Design review of the part built by this model. Coordinates are the model's own, in mm. A direction names the side the tool comes from. Round coordinates to 2 decimals unless told otherwise and drop trailing zeros. Order: outer loops, then holes, each group sorted by start corner. A loop starts at its lowest first (then second) coordinate and runs counter-clockwise, first axis right, second up.
from build123d import *

# Parameters (mm, degrees)
F0_W      = 19
F0_H      = 19
F1_DEPTH  = 19
F3_DEPTH  = 1
F4_R      = 1
F5_DEPTH  = 1
F6_R      = 1
F7_DEPTH  = 1
F8_R      = 1
F9_DEPTH  = 1
F10_R     = 1
F11_DEPTH = 1
F12_R     = 1
F13_DEPTH = 1
F14_R     = 1


with BuildPart() as f1:
    # F0 (on Top) → F1 (new body)
    with BuildSketch(Plane.XY):
        with Locations((-9.5, 9.5)):
            Rectangle(F0_W, F0_H)
    extrude(amount=F1_DEPTH)

    # F2 (on face) → F3 (cut)
    with BuildSketch(Plane.XY.offset(19)):
        with BuildLine():
            ThreePointArc((-10.6875, 9.818189666), (-11.556810334, 10.6875), (-11.875, 11.875))
            Line((-11.875, 11.875), (-11.875, 7.125))
            ThreePointArc((-11.875, 7.125), (-11.556810334, 8.3125), (-10.6875, 9.181810334))
            Line((-10.6875, 9.181810334), (-10.6875, 9.818189666))
        make_face()
        with BuildLine():
            ThreePointArc((-10.6875, 13.931810334), (-11.556810334, 13.0625), (-11.875, 11.875))
            ThreePointArc((-11.875, 11.875), (-11.556810334, 10.6875), (-10.6875, 9.818189666))
            Line((-10.6875, 9.818189666), (-10.6875, 11.875))
            Line((-10.6875, 11.875), (-10.6875, 13.931810334))
        make_face()
        with BuildLine():
            ThreePointArc((-7.125, 11.875), (-8.3125, 13.931810334), (-10.6875, 13.931810334))
            Line((-10.6875, 13.931810334), (-10.6875, 11.875))
            Line((-10.6875, 11.875), (-10.6875, 9.818189666))
            ThreePointArc((-10.6875, 9.818189666), (-10.1146952321, 9.5809261626), (-9.5, 9.5))
            ThreePointArc((-9.5, 9.5), (-7.8206213947, 10.1956213947), (-7.125, 11.875))
        make_face()
        with BuildLine():
            ThreePointArc((-8.3125, 11.875), (-9.5, 10.6875), (-10.6875, 11.875))
            ThreePointArc((-10.6875, 11.875), (-9.5, 13.0625), (-8.3125, 11.875))
        make_face(mode=Mode.SUBTRACT)
        with BuildLine():
            ThreePointArc((-9.5, 9.5), (-10.1146952321, 9.4190738374), (-10.6875, 9.181810334))
            Line((-10.6875, 9.181810334), (-10.6875, 7.125))
            Line((-10.6875, 7.125), (-10.6875, 5.068189666))
            ThreePointArc((-10.6875, 5.068189666), (-8.3125, 5.068189666), (-7.125, 7.125))
            ThreePointArc((-7.125, 7.125), (-7.8206213947, 8.8043786053), (-9.5, 9.5))
        make_face()
        with BuildLine():
            ThreePointArc((-8.3125, 7.125), (-9.5, 5.9375), (-10.6875, 7.125))
            ThreePointArc((-10.6875, 7.125), (-9.5, 8.3125), (-8.3125, 7.125))
        make_face(mode=Mode.SUBTRACT)
        with BuildLine():
            ThreePointArc((-10.6875, 9.181810334), (-11.556810334, 8.3125), (-11.875, 7.125))
            ThreePointArc((-11.875, 7.125), (-11.556810334, 5.9375), (-10.6875, 5.068189666))
            Line((-10.6875, 5.068189666), (-10.6875, 7.125))
            Line((-10.6875, 7.125), (-10.6875, 9.181810334))
        make_face()
        with BuildLine():
            ThreePointArc((-9.5, 9.5), (-10.1146952321, 9.5809261626), (-10.6875, 9.818189666))
            Line((-10.6875, 9.818189666), (-10.6875, 9.181810334))
            ThreePointArc((-10.6875, 9.181810334), (-10.1146952321, 9.4190738374), (-9.5, 9.5))
        make_face()
        with BuildLine():
            ThreePointArc((-10.6875, 5.068189666), (-11.556810334, 5.9375), (-11.875, 7.125))
            Line((-11.875, 7.125), (-11.875, 4.75))
            Line((-11.875, 4.75), (-10.6875, 4.75))
            Line((-10.6875, 4.75), (-10.6875, 5.068189666))
        make_face()
        with BuildLine():
            Line((-10.6875, 14.25), (-11.875, 14.25))
            Line((-11.875, 14.25), (-11.875, 11.875))
            ThreePointArc((-11.875, 11.875), (-11.556810334, 13.0625), (-10.6875, 13.931810334))
            Line((-10.6875, 13.931810334), (-10.6875, 14.25))
        make_face()
    extrude(amount=-F3_DEPTH, mode=Mode.SUBTRACT)

    # F4 (on face) → F5 (cut)
    with BuildSketch(Plane.XZ):
        with Locations((-14.25, 14.25)):
            Circle(F4_R)
        with Locations((-4.75, 4.75)):
            Circle(F4_R)
    extrude(amount=-F5_DEPTH, mode=Mode.SUBTRACT)

    # F6 (on face) → F7 (cut)
    with BuildSketch(Plane(origin=(0, 0, 0), x_dir=(1, 0, 0), z_dir=(0, 0, -1))):
        with Locations((-14.25, -4.75)):
            Circle(F6_R)
        with Locations((-9.5, -9.5)):
            Circle(F6_R)
        with Locations((-4.75, -4.75)):
            Circle(F6_R)
        with Locations((-4.75, -14.25)):
            Circle(F6_R)
        with Locations((-14.25, -14.25)):
            Circle(F6_R)
    extrude(amount=-F7_DEPTH, mode=Mode.SUBTRACT)

    # F8 (on face) → F9 (cut)
    with BuildSketch(Plane(origin=(0, 19, 0), x_dir=(-1, 0, 0), z_dir=(0, 1, 0))):
        with Locations((4.75, 14.25)):
            Circle(F8_R)
        with Locations((4.75, 9.5)):
            Circle(F8_R)
        with Locations((4.75, 4.75)):
            Circle(F8_R)
        with Locations((14.25, 4.75)):
            Circle(F8_R)
        with Locations((14.25, 9.5)):
            Circle(F8_R)
        with Locations((14.25, 14.25)):
            Circle(F8_R)
    extrude(amount=-F9_DEPTH, mode=Mode.SUBTRACT)

    # F10 (on face) → F11 (cut)
    with BuildSketch(Plane.YZ):
        with Locations((4.75, 4.75)):
            Circle(F10_R)
        with Locations((9.5, 9.5)):
            Circle(F10_R)
        with Locations((14.25, 14.25)):
            Circle(F10_R)
    extrude(amount=-F11_DEPTH, mode=Mode.SUBTRACT)

    # F12 (on face) → F13 (cut)
    with BuildSketch(Plane(origin=(-19, 0, 0), x_dir=(0, -1, 0), z_dir=(-1, 0, 0))):
        with Locations((-14.25, 14.25)):
            Circle(F12_R)
        with Locations((-4.75, 14.25)):
            Circle(F12_R)
        with Locations((-14.25, 4.75)):
            Circle(F12_R)
        with Locations((-4.75, 4.75)):
            Circle(F12_R)
    extrude(amount=-F13_DEPTH, mode=Mode.SUBTRACT)

    # F14
    f14_edges = [f1.edges().sort_by_distance(p)[0] for p in [
        (0, 9.5, 19),
        (-9.5, 19, 19),
        (-9.5, 0, 19),
        (-19, 9.5, 19),
        (-19, 0, 9.5),
        (-19, 19, 9.5),
        (0, 19, 9.5),
        (0, 0, 9.5),
        (-9.5, 0, 0),
        (-9.5, 19, 0),
        (-19, 9.5, 0),
        (0, 9.5, 0),
    ]]
    fillet(f14_edges, radius=F14_R)


solid = f1.part
1) To check wall thickness, follow line 1 along X through (y, z) = (14.25, 0.3); line 2 along X through (y, z) = (4.75, 0.35); line 3 along Z through (x, y) = (-18.65, 14.25). State the ranges of each line that lie inside material, in increasing order.
Results:
line 1: x = -18.71 to -15.25, -13.25 to -5.75, -3.75 to -0.29
line 2: x = -18.76 to -15.25, -13.25 to -5.75, -3.75 to -0.24
line 3: z = 0.24 to 3.75, 5.75 to 13.25, 15.25 to 18.76
2) Take a section at A-A on x = -11. Give the boundary of the cut face in (y, z), plus the area to 3 significant figures.
Results:
outline: (0, 1) arc R1 ccw to (1, 0) - (18, 0) arc R1 ccw to (19, 1) - (19, 18) arc R1 ccw to (18, 19) - (14.25, 19) - (14.25, 18) - (4.75, 18) - (4.75, 19) - (1, 19) arc R1 ccw to (0, 18) - close
area: 351 mm2
3) Clearance check with flat-ended pins moving along their axes: P1, Ø1.2, axis at x = -14.25, z = 9.5, coming from the +Y side; P2, Ø1, axis at y = 4.5, z = 5, coming from the +X side; P3, Ø0.6, axis at x = -14.5, z = 14, coming from the -Y side. State where each tip first meets the part, or that it passes through.
Results:
P1: stops at y = 18
P2: stops at x = -1
P3: stops at y = 1
4) The part is to be moulded in two halves that separate along X. For faces 1 (the face through (-13.79, 0.49, 13.36)), 2 (the face through (-1, 5, 5)), 3 (the face through (-18.507, 13.296, 5.05)), 4 (the face through (-11.3, 14.25, 18.5)), say which applies: released by +X, released by -X, zero draft, split by the parting line, or undercut.
Results:
face 1: undercut
face 2: released by +X
face 3: zero draft
face 4: undercut
5) For faces 5 (the face through (-14, 18, 5)), 6 (the face through (-0.49, 9.37, 10.49)), 7 (the face through (-18.51, 13.79, 13.36)), 8 (the face through (-13.79, 15.14, 0.49)), list the 3-axis set-ups (+Z, -Z, +X, -X, +Y, -Y) from which the entire face can be reached by the end or side of a thin tool; tool diameter is ignored.
Results:
face 5: +Y
face 6: +X
face 7: -X
face 8: -Z
6) Take a section at B-B on z = 9.5. Give the boundary of the cut face in (x, y).
Results:
outline: (-19, 1) arc R1 ccw to (-18, 0) - (-1, 0) arc R1 ccw to (0, 1) - (0, 8.5) - (-1, 8.5) - (-1, 10.5) - (0, 10.5) - (0, 18) arc R1 ccw to (-1, 19) - (-3.75, 19) - (-3.75, 18) - (-5.75, 18) - (-5.75, 19) - (-13.25, 19) - (-13.25, 18) - (-15.25, 18) - (-15.25, 19) - (-18, 19) arc R1 ccw to (-19, 18) - close
